Check sheet for the modelled part. Datum: model origin and axes. Units: mm. Face numbers are marked on the shaded views. A direction names the side the tool comes from. Round coordinates to 2 decimals unless told otherwise and drop trailing zeros. Order: outer loops, then holes, each group sorted by start corner. A loop starts at its lowest first (then second) coordinate and runs counter-clockwise, first axis right, second up. Notation, with made-up numbers: (22.25, 35) -> (39.25, 35) arc R12 ccw to (39.25, 57) -> close; hole circle Ø2 at (-30.5, 2). An arc over 180 degrees is marked (long way). Answer in a Markdown table with one row per item.
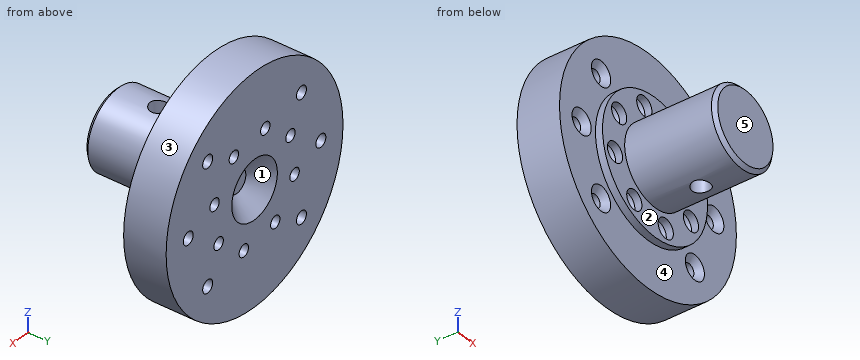
from build123d import *

# Parameters (mm, degrees)
SKETCH1_R                                            = 32
SKETCH1_R_2                                          = 8.25
BOSS_EXTRUDE1_DEPTH                                  = 12
CSK_FOR_M3_HEX_SOCKET_COUNTERSUNK_HEAD_S_D           = 3.4
CSK_FOR_M3_HEX_SOCKET_COUNTERSUNK_HEAD_S_CSINK_D     = 5.5
CSK_FOR_M3_HEX_SOCKET_COUNTERSUNK_HEAD_S_CSINK_ANGLE = 90
CSK_FOR_M3_HEX_SOCKET_COUNTERSUNK_HE_2_D             = 3.6
CSK_FOR_M3_HEX_SOCKET_COUNTERSUNK_HE_2_CSINK_D       = 6.94
CSK_FOR_M3_HEX_SOCKET_COUNTERSUNK_HE_2_CSINK_ANGLE   = 90
BOSS_EXTRUDE2_DEPTH                                  = 27.5
BOSS_EXTRUDE2_DEPTH_BACK                             = 7
SKETCH10_R                                           = 19
SKETCH10_R_2                                         = 2.75
CUT_EXTRUDE2_START                                   = -25.5
SKETCH11_R                                           = 19
SKETCH11_R_2                                         = 11
CUT_EXTRUDE2_DEPTH                                   = 25.5
CHAMFER1_SIZE                                        = 5
CHAMFER2_SIZE                                        = 1
F_4_2_4_2_DIAMETER_HOLE1_D                           = 4.2
SKETCH27_R                                           = 2.5
CUT_EXTRUDE3_DEPTH                                   = 8.5
CUT_EXTRUDE4_START                                   = 8.5
SKETCH28_R                                           = 2.5
CUT_EXTRUDE4_DEPTH                                   = 8.5


with BuildPart() as part:
    # Sketch1 → Boss-Extrude1 (new body)
    with BuildSketch(Plane(origin=(0, 0, 0), x_dir=(1, 0, 0), z_dir=(0, 1, 0))):
        with Locations(Location((0, 0, 0), (0, 0, 270))):
            Circle(SKETCH1_R)
        with Locations(Location((0, 0, 0), (0, 0, 270))):
            Circle(SKETCH1_R_2, mode=Mode.SUBTRACT)
    extrude(amount=BOSS_EXTRUDE1_DEPTH)

    # CSK for M3 Hex Socket Countersunk Head S (through all)
    with Locations(Plane.XZ):
        with Locations((3.882285677, -14.488887394), (12.990381057, -7.5), (14.488887394, 3.882285677), (7.5, 12.990381057), (-3.882285677, 14.488887394), (-12.990381057, 7.5), (-14.488887394, -3.882285677), (-7.5, -12.990381057)):
            CounterSinkHole(CSK_FOR_M3_HEX_SOCKET_COUNTERSUNK_HEAD_S_D / 2, CSK_FOR_M3_HEX_SOCKET_COUNTERSUNK_HEAD_S_CSINK_D / 2, counter_sink_angle=CSK_FOR_M3_HEX_SOCKET_COUNTERSUNK_HEAD_S_CSINK_ANGLE)

    # CSK for M3 Hex Socket Countersunk He 2 (through all)
    with Locations(Plane(origin=(0, 0, 0), x_dir=(-1, 0, 0), z_dir=(0, -1, 0))):
        with Locations((-16.970562748, -16.970562748), (-24, 0), (-16.970562748, 16.970562748), (16.970562748, 16.970562748), (24, 0), (16.970562748, -16.970562748)):
            CounterSinkHole(CSK_FOR_M3_HEX_SOCKET_COUNTERSUNK_HE_2_D / 2, CSK_FOR_M3_HEX_SOCKET_COUNTERSUNK_HE_2_CSINK_D / 2, counter_sink_angle=CSK_FOR_M3_HEX_SOCKET_COUNTERSUNK_HE_2_CSINK_ANGLE)

    # Sketch10 → Boss-Extrude2 (add, two sides: drawn at the far end of the back side and taken through both)
    with BuildSketch(Plane.XZ.offset(-BOSS_EXTRUDE2_DEPTH_BACK)):
        with Locations(Location((0, 0, 0), (0, 0, 270))):
            Circle(SKETCH10_R)
        with Locations(Location((7.5, 12.990381057, 0), (0, 0, 270))):
            Circle(SKETCH10_R_2, mode=Mode.SUBTRACT)
        with Locations(Location((14.488887394, 3.882285677, 0), (0, 0, 270))):
            Circle(SKETCH10_R_2, mode=Mode.SUBTRACT)
        with Locations(Location((12.990381057, -7.5, 0), (0, 0, 270))):
            Circle(SKETCH10_R_2, mode=Mode.SUBTRACT)
        with Locations(Location((3.882285677, -14.488887394, 0), (0, 0, 270))):
            Circle(SKETCH10_R_2, mode=Mode.SUBTRACT)
        with Locations(Location((-7.5, -12.990381057, 0), (0, 0, 270))):
            Circle(SKETCH10_R_2, mode=Mode.SUBTRACT)
        with Locations(Location((-14.488887394, -3.882285677, 0), (0, 0, 270))):
            Circle(SKETCH10_R_2, mode=Mode.SUBTRACT)
        with Locations(Location((-12.990381057, 7.5, 0), (0, 0, 270))):
            Circle(SKETCH10_R_2, mode=Mode.SUBTRACT)
        with Locations(Location((-3.882285677, 14.488887394, 0), (0, 0, 270))):
            Circle(SKETCH10_R_2, mode=Mode.SUBTRACT)
    extrude(amount=BOSS_EXTRUDE2_DEPTH + BOSS_EXTRUDE2_DEPTH_BACK)

    # Sketch11 → Cut-Extrude2 (cut)
    with BuildSketch(Plane.XZ.offset(27.5).offset(CUT_EXTRUDE2_START)):
        with Locations(Location((0, 0, 0), (0, 0, 270))):
            Circle(SKETCH11_R)
        with Locations(Location((0, 0, 0), (0, 0, 270))):
            Circle(SKETCH11_R_2, mode=Mode.SUBTRACT)
    extrude(amount=CUT_EXTRUDE2_DEPTH, mode=Mode.SUBTRACT)

    # Chamfer1
    chamfer1_edges = [part.edges().sort_by_distance(p)[0] for p in [
        (0, 7, -8.25),
    ]]
    chamfer(chamfer1_edges, length=CHAMFER1_SIZE - 0.0001)  # a hair under: the kernel refuses the full size

    # Chamfer2
    chamfer2_edges = [part.edges().sort_by_distance(p)[0] for p in [
        (0, -27.5, 11),
    ]]
    chamfer(chamfer2_edges, length=CHAMFER2_SIZE)

    # Ø4.2 (4.2) Diameter Hole1 (through all)
    with Locations(Plane.XY.offset(15)):
        with Locations((0, -15)):
            Hole(F_4_2_4_2_DIAMETER_HOLE1_D / 2)

    # Sketch27 → Cut-Extrude3 (cut)
    with BuildSketch(Plane.XY.offset(15)):
        with Locations((0, -15)):
            Circle(SKETCH27_R)
    extrude(amount=-CUT_EXTRUDE3_DEPTH, mode=Mode.SUBTRACT)

    # Sketch28 → Cut-Extrude4 (cut)
    with BuildSketch(Plane.XY.offset(-15).offset(CUT_EXTRUDE4_START)):
        with Locations((0, -15)):
            Circle(SKETCH28_R)
    extrude(amount=-CUT_EXTRUDE4_DEPTH, mode=Mode.SUBTRACT)


solid = part.part
Item 1: Depth check by flat-ended pin: P1, Ø4.5, axis at x = -16.97, z = 16.97, coming from the -Y side; P2, Ø8, axis at y = -14, z = -13.5, coming from the -X side; P3, Ø5, axis at x = -5, y = -13, coming from the +Z side. Enter the tip coordinate at first touch or a pass-through.
Result sheet:
| item | result |
|---|---|
| P1 | stops at y = 1.22 |
| P2 | stops at x = -5.55 |
| P3 | stops at z = 10.71 |
Item 2: Cross-section at D-D (x = -24). Record the boundary of the cut face in (y, z).
Result sheet:
| item | result |
|---|---|
| outline | (0, -21.17) -> (12, -21.17) -> (12, -1.8) -> (1.67, -1.8) -> (0, -3.47) -> close; (0, 3.47) -> (1.67, 1.8) -> (12, 1.8) -> (12, 21.17) -> (0, 21.17) -> close |
Item 3: Cross-section at A-A (z = 0). State how many separate pieces and enclosed holes the cut face has, and give its area (3 significant figures).
Result sheet:
| item | result |
|---|---|
| separate pieces | 3 |
| enclosed holes | 1 |
| area | 1,240 mm^2 |
Item 4: Cross-section at C-C (y = -15). Record the boundary of the cut face in (x, z), and give its area (3 significant figures).
Result sheet:
| item | result |
|---|---|
| outline | (-2.5, -10.71) -> (-2.5, -6.5) -> (-2.1, -6.5) -> (-2.1, 6.5) -> (-2.5, 6.5) -> (-2.5, 10.71) arc R11 ccw to start; (2.1, -6.5) -> (2.5, -6.5) -> (2.5, -10.71) arc R11 ccw to (2.5, 10.71) -> (2.5, 6.5) -> (2.1, 6.5) -> close |
| area | 281 mm^2 |
Item 5: Set-up check for the marked faces 4 and 5: record each of +Z, -Z, +X, -X, +Y, -Y from which the full face is reachable in a straight line by a thin tool's end or side.
Result sheet:
| item | result |
|---|---|
| face 4 | -Y |
| face 5 | +Z, -Z, +X, -X, -Y |
Item 6: Scan lines: line 1 (X direction, y = 5, z = 17.5); line 2 (Y direction, x = 0, z = 9.65); line 3 (X direction, y = 10, z = 4). Record each from-to range of solid material in increasing order. Write a range as [from, to].
Result sheet:
| item | result |
|---|---|
| line 1 | x = [-26.79, -18.69], [-15.25, 15.25], [18.69, 26.79] |
| line 2 | y = [-27.5, -17.5], [-12.5, 12] |
| line 3 | x = [-31.75, -4.8], [4.8, 12.79], [16.18, 31.75] |
Item 7: Mould release check, pull along Z, two halves, no side actions. Record for the marked faces 1, 2 and 3: pulls with the +Z half, pulls with the -Z half, needs draft (parallel to the pull), parting line crosses it, or undercut.
Result sheet:
| item | result |
|---|---|
| face 1 | undercut |
| face 2 | needs draft |
| face 3 | parting line crosses it |
